Source: CAD feature listing. Evaluate the final solid. Frame: model axes, mm. Coordinates: 2 decimals unless noted, no trailing zeros. One line per item, written item: value. Start each with the question number.
Item 1: Pin query (flat end, axial travel): P1, Ø1, axis at y = 41, z = 4.5, coming from the +X side; P2, Ø11.5, axis at x = -61.34, y = 16.44, coming from the -Z side; P3, Ø2, axis at y = 43, z = 4.5, coming from the +X side. Return the tip coordinate at first contact, or that it passes through.
Item 2: Mould query, pull axis Y, two halves, no side actions, for faces 1 (the cylindrical face through (67.2, -18.87, 3.13)), 2 (the cylindrical face through (78.612, -32.565, 3.131)), 3 (the cylindrical face through (-22.025, -99.184, 3.131)). Classes: released by +Y, released by -Y, zero draft, split by the parting line, or undercut.
Item 3: Ray query, L1, parallel to Y at x = -24.5, z = 4.75; L2, parallel to X at y = -23.5, z = 3.25; L3, parallel to Y at x = -11, z = 3. Return the intervals inside material, ascending. Write a range as from..to.
Item 4: Cut plane A-A, the plane z = 3.75. State how many separate pieces and enclosed holes the cut face has, then the cut area to 3 significant figures.
```python
from build123d import *

# Parameters (mm, degrees)
SKETCH1_R                   = 101.6
SKETCH1_R_2                 = 6.35
SKETCH1_R_3                 = 7.62
SKETCH1_R_4                 = 8.382
BOSS_EXTRUDE1_DEPTH         = 6.35
F_1_4_CLEARANCE_HOLE1_D     = 6.7564
F_1_4_CLEARANCE_HOLE1_DEPTH = 9.652
F_1_4_CLEARANCE_HOLE1_TIP   = 2.029827343


with BuildPart() as part:
    # Sketch1 → Boss-Extrude1 (new body)
    with BuildSketch(Plane.XY):
        Circle(SKETCH1_R)
        with Locations((0, 63.5)):
            Circle(SKETCH1_R_2, mode=Mode.SUBTRACT)
        with Locations((16.435009364, 61.336289969)):
            Circle(SKETCH1_R_2, mode=Mode.SUBTRACT)
        with Locations((31.75, 54.99261314)):
            Circle(SKETCH1_R_2, mode=Mode.SUBTRACT)
        with Locations((44.901280605, 44.901280605)):
            Circle(SKETCH1_R_2, mode=Mode.SUBTRACT)
        with Locations((54.99261314, 31.75)):
            Circle(SKETCH1_R_2, mode=Mode.SUBTRACT)
        with Locations((61.336289969, 16.435009364)):
            Circle(SKETCH1_R_2, mode=Mode.SUBTRACT)
        with Locations((63.5, 0)):
            Circle(SKETCH1_R_2, mode=Mode.SUBTRACT)
        with Locations((61.336289969, -16.435009364)):
            Circle(SKETCH1_R_2, mode=Mode.SUBTRACT)
        with Locations((54.99261314, -31.75)):
            Circle(SKETCH1_R_2, mode=Mode.SUBTRACT)
        with Locations((44.901280605, -44.901280605)):
            Circle(SKETCH1_R_2, mode=Mode.SUBTRACT)
        with Locations((31.75, -54.99261314)):
            Circle(SKETCH1_R_2, mode=Mode.SUBTRACT)
        with Locations((16.435009364, -61.336289969)):
            Circle(SKETCH1_R_2, mode=Mode.SUBTRACT)
        with Locations((0, -63.5)):
            Circle(SKETCH1_R_2, mode=Mode.SUBTRACT)
        with Locations((-16.435009364, -61.336289969)):
            Circle(SKETCH1_R_2, mode=Mode.SUBTRACT)
        with Locations((-31.75, -54.99261314)):
            Circle(SKETCH1_R_2, mode=Mode.SUBTRACT)
        with Locations((-44.901280605, -44.901280605)):
            Circle(SKETCH1_R_2, mode=Mode.SUBTRACT)
        with Locations((-54.99261314, -31.75)):
            Circle(SKETCH1_R_2, mode=Mode.SUBTRACT)
        with Locations((-61.336289969, -16.435009364)):
            Circle(SKETCH1_R_2, mode=Mode.SUBTRACT)
        with Locations((-63.5, 0)):
            Circle(SKETCH1_R_2, mode=Mode.SUBTRACT)
        with Locations((-61.336289969, 16.435009364)):
            Circle(SKETCH1_R_2, mode=Mode.SUBTRACT)
        with Locations((-54.99261314, 31.75)):
            Circle(SKETCH1_R_2, mode=Mode.SUBTRACT)
        with Locations((-44.901280605, 44.901280605)):
            Circle(SKETCH1_R_2, mode=Mode.SUBTRACT)
        with Locations((-31.75, 54.99261314)):
            Circle(SKETCH1_R_2, mode=Mode.SUBTRACT)
        with Locations((-16.435009364, 61.336289969)):
            Circle(SKETCH1_R_2, mode=Mode.SUBTRACT)
        with Locations((10.111864111, 76.807233411)):
            Circle(SKETCH1_R_3, mode=Mode.SUBTRACT)
        with Locations((29.646485505, 71.572947384)):
            Circle(SKETCH1_R_3, mode=Mode.SUBTRACT)
        with Locations((47.160747905, 61.461083272)):
            Circle(SKETCH1_R_3, mode=Mode.SUBTRACT)
        with Locations((61.461083272, 47.160747905)):
            Circle(SKETCH1_R_3, mode=Mode.SUBTRACT)
        with Locations((71.572947384, 29.646485505)):
            Circle(SKETCH1_R_3, mode=Mode.SUBTRACT)
        with Locations((76.807233411, 10.111864111)):
            Circle(SKETCH1_R_3, mode=Mode.SUBTRACT)
        with Locations((76.807233411, -10.111864111)):
            Circle(SKETCH1_R_3, mode=Mode.SUBTRACT)
        with Locations((71.572947384, -29.646485505)):
            Circle(SKETCH1_R_3, mode=Mode.SUBTRACT)
        with Locations((61.461083272, -47.160747905)):
            Circle(SKETCH1_R_3, mode=Mode.SUBTRACT)
        with Locations((47.160747905, -61.461083272)):
            Circle(SKETCH1_R_3, mode=Mode.SUBTRACT)
        with Locations((29.646485505, -71.572947384)):
            Circle(SKETCH1_R_3, mode=Mode.SUBTRACT)
        with Locations((10.111864111, -76.807233411)):
            Circle(SKETCH1_R_3, mode=Mode.SUBTRACT)
        with Locations((-10.111864111, -76.807233411)):
            Circle(SKETCH1_R_3, mode=Mode.SUBTRACT)
        with Locations((-29.646485505, -71.572947384)):
            Circle(SKETCH1_R_3, mode=Mode.SUBTRACT)
        with Locations((-47.160747905, -61.461083272)):
            Circle(SKETCH1_R_3, mode=Mode.SUBTRACT)
        with Locations((-61.461083272, -47.160747905)):
            Circle(SKETCH1_R_3, mode=Mode.SUBTRACT)
        with Locations((-71.572947384, -29.646485505)):
            Circle(SKETCH1_R_3, mode=Mode.SUBTRACT)
        with Locations((-76.807233411, -10.111864111)):
            Circle(SKETCH1_R_3, mode=Mode.SUBTRACT)
        with Locations((-76.807233411, 10.111864111)):
            Circle(SKETCH1_R_3, mode=Mode.SUBTRACT)
        with Locations((-71.572947384, 29.646485505)):
            Circle(SKETCH1_R_3, mode=Mode.SUBTRACT)
        with Locations((-61.461083272, 47.160747905)):
            Circle(SKETCH1_R_3, mode=Mode.SUBTRACT)
        with Locations((-47.160747905, 61.461083272)):
            Circle(SKETCH1_R_3, mode=Mode.SUBTRACT)
        with Locations((-29.646485505, 71.572947384)):
            Circle(SKETCH1_R_3, mode=Mode.SUBTRACT)
        with Locations((-10.111864111, 76.807233411)):
            Circle(SKETCH1_R_3, mode=Mode.SUBTRACT)
        with Locations((0, 91.948)):
            Circle(SKETCH1_R_4, mode=Mode.SUBTRACT)
        with Locations((23.797893559, 88.814947876)):
            Circle(SKETCH1_R_4, mode=Mode.SUBTRACT)
        with Locations((45.974, 79.629303827)):
            Circle(SKETCH1_R_4, mode=Mode.SUBTRACT)
        with Locations((65.017054317, 65.017054317)):
            Circle(SKETCH1_R_4, mode=Mode.SUBTRACT)
        with Locations((79.629303827, 45.974)):
            Circle(SKETCH1_R_4, mode=Mode.SUBTRACT)
        with Locations((88.814947876, 23.797893559)):
            Circle(SKETCH1_R_4, mode=Mode.SUBTRACT)
        with Locations((91.948, 0)):
            Circle(SKETCH1_R_4, mode=Mode.SUBTRACT)
        with Locations((88.814947876, -23.797893559)):
            Circle(SKETCH1_R_4, mode=Mode.SUBTRACT)
        with Locations((79.629303827, -45.974)):
            Circle(SKETCH1_R_4, mode=Mode.SUBTRACT)
        with Locations((65.017054317, -65.017054317)):
            Circle(SKETCH1_R_4, mode=Mode.SUBTRACT)
        with Locations((45.974, -79.629303827)):
            Circle(SKETCH1_R_4, mode=Mode.SUBTRACT)
        with Locations((23.797893559, -88.814947876)):
            Circle(SKETCH1_R_4, mode=Mode.SUBTRACT)
        with Locations((0, -91.948)):
            Circle(SKETCH1_R_4, mode=Mode.SUBTRACT)
        with Locations((-23.797893559, -88.814947876)):
            Circle(SKETCH1_R_4, mode=Mode.SUBTRACT)
        with Locations((-45.974, -79.629303827)):
            Circle(SKETCH1_R_4, mode=Mode.SUBTRACT)
        with Locations((-65.017054317, -65.017054317)):
            Circle(SKETCH1_R_4, mode=Mode.SUBTRACT)
        with Locations((-79.629303827, -45.974)):
            Circle(SKETCH1_R_4, mode=Mode.SUBTRACT)
        with Locations((-88.814947876, -23.797893559)):
            Circle(SKETCH1_R_4, mode=Mode.SUBTRACT)
        with Locations((-91.948, 0)):
            Circle(SKETCH1_R_4, mode=Mode.SUBTRACT)
        with Locations((-88.814947876, 23.797893559)):
            Circle(SKETCH1_R_4, mode=Mode.SUBTRACT)
        with Locations((-79.629303827, 45.974)):
            Circle(SKETCH1_R_4, mode=Mode.SUBTRACT)
        with Locations((-65.017054317, 65.017054317)):
            Circle(SKETCH1_R_4, mode=Mode.SUBTRACT)
        with Locations((-45.974, 79.629303827)):
            Circle(SKETCH1_R_4, mode=Mode.SUBTRACT)
        with Locations((-23.797893559, 88.814947876)):
            Circle(SKETCH1_R_4, mode=Mode.SUBTRACT)
        with BuildLine():
            ThreePointArc((-28.409048011, -3.727209563), (-28.652505999, 0), (-28.409048011, 3.727209563))
            ThreePointArc((-28.409048011, 3.727209563), (-28.828314509, 5.763343193), (-30.417415023, 7.10363574))
            ThreePointArc((-30.417415023, 7.10363574), (-36.698388219, 36.698388219), (-7.10363574, 30.417415023))
            ThreePointArc((-7.10363574, 30.417415023), (-5.763343193, 28.828314509), (-3.727209563, 28.409048011))
            ThreePointArc((-3.727209563, 28.409048011), (0, 28.652505999), (3.727209563, 28.409048011))
            ThreePointArc((3.727209563, 28.409048011), (5.763343193, 28.828314509), (7.10363574, 30.417415023))
            ThreePointArc((7.10363574, 30.417415023), (36.698388219, 36.698388219), (30.417415023, 7.10363574))
            ThreePointArc((30.417415023, 7.10363574), (28.828314509, 5.763343193), (28.409048011, 3.727209563))
            ThreePointArc((28.409048011, 3.727209563), (28.652505999, 0), (28.409048011, -3.727209563))
            ThreePointArc((28.409048011, -3.727209563), (28.828314509, -5.763343193), (30.417415023, -7.10363574))
            ThreePointArc((30.417415023, -7.10363574), (36.698388219, -36.698388219), (7.10363574, -30.417415023))
            ThreePointArc((7.10363574, -30.417415023), (5.763343193, -28.828314509), (3.727209563, -28.409048011))
            ThreePointArc((3.727209563, -28.409048011), (0, -28.652505999), (-3.727209563, -28.409048011))
            ThreePointArc((-3.727209563, -28.409048011), (-5.763343193, -28.828314509), (-7.10363574, -30.417415023))
            ThreePointArc((-7.10363574, -30.417415023), (-36.698388219, -36.698388219), (-30.417415023, -7.10363574))
            ThreePointArc((-30.417415023, -7.10363574), (-28.828314509, -5.763343193), (-28.409048011, -3.727209563))
        make_face(mode=Mode.SUBTRACT)
    extrude(amount=BOSS_EXTRUDE1_DEPTH)

    # 1/4 Clearance Hole1
    with Locations(Plane(origin=(0, 34.29, 6.35), x_dir=(1, 0, 0), z_dir=(0, 0, 1))):
        with Locations((0, 0), (-34.29, -34.29), (34.29, -34.29), (0, -68.58)):
            Hole(F_1_4_CLEARANCE_HOLE1_D / 2, depth=F_1_4_CLEARANCE_HOLE1_DEPTH)
            with Locations((0, 0, -(F_1_4_CLEARANCE_HOLE1_DEPTH + F_1_4_CLEARANCE_HOLE1_TIP / 2))):  # 118° drill point
                Cone(0, F_1_4_CLEARANCE_HOLE1_D / 2, F_1_4_CLEARANCE_HOLE1_TIP, mode=Mode.SUBTRACT)


solid = part.part
```
From the geometry:
1. P1: stops at x = 93.18
1. P2: passes through
1. P3: stops at x = 92.51
2. face 1: undercut
2. face 2: undercut
2. face 3: split by the parting line
3. L1: y = -98.6..-97.17, -80.46..-77.19, -65.95..-41.97, 41.97..65.95, 77.19..80.46, 97.17..98.6
3. L2: x = -98.84..-97.19, -80.44..-76.08, -67.07..-41.98, 41.98..67.07, 76.08..80.44, 97.19..98.84
3. L3: y = -101..-84.38, -69.24..-64.62, -58.05..-36.51, 36.51..58.05, 64.62..69.24, 84.38..101
4. separate pieces: 1
4. enclosed holes: 77
4. area: 14,000 mm²
